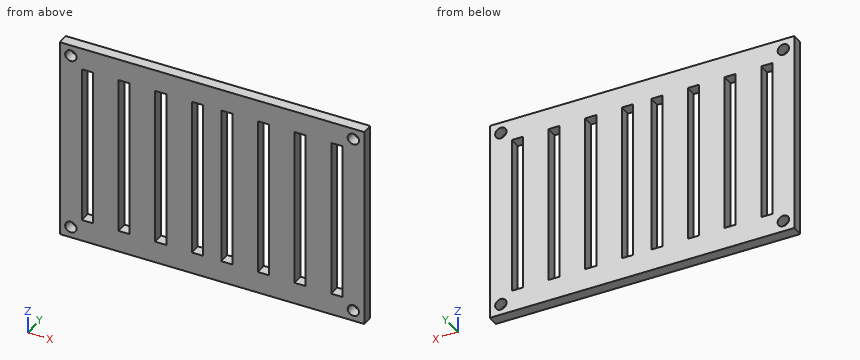
from build123d import *

# Parameters (mm, degrees)
SKETCH_1_W          = 83
SKETCH_1_H          = 56
SKETCH_1_R          = 1.55
EXTRUDE_1_DEPTH     = 3
SKETCH_3_W          = 3
SKETCH_3_H          = 44
CUT_EXTRUDE_1_DEPTH = 51.152268144


with BuildPart() as part:
    # ｽｹｯﾁ1 → ﾎﾞｽ - 押し出し1 (new body)
    with BuildSketch(Plane(origin=(0, 0, 0), x_dir=(1, 0, 0), z_dir=(0, 1, 0))):
        Rectangle(SKETCH_1_W, SKETCH_1_H)
        with Locations(Location((-38.5, 25, 0), (0, 0, 270))):
            Circle(SKETCH_1_R, mode=Mode.SUBTRACT)
        with Locations(Location((38.5, 25, 0), (0, 0, 270))):
            Circle(SKETCH_1_R, mode=Mode.SUBTRACT)
        with Locations(Location((38.5, -25, 0), (0, 0, 270))):
            Circle(SKETCH_1_R, mode=Mode.SUBTRACT)
        with Locations(Location((-38.5, -25, 0), (0, 0, 270))):
            Circle(SKETCH_1_R, mode=Mode.SUBTRACT)
    extrude(amount=EXTRUDE_1_DEPTH)

    # ｽｹｯﾁ3 → ｶｯﾄ - 押し出し1 (cut, through all)
    with BuildSketch(Plane(origin=(0, 3, 0), x_dir=(1, 0, 0), z_dir=(0, 1, 0))):
        with Locations((-34, 0)):
            Rectangle(SKETCH_3_W, SKETCH_3_H)
        with Locations((-24, 0)):
            Rectangle(SKETCH_3_W, SKETCH_3_H)
        with Locations((-14, 0)):
            Rectangle(SKETCH_3_W, SKETCH_3_H)
        with Locations((-4, 0)):
            Rectangle(SKETCH_3_W, SKETCH_3_H)
        with Locations((4, 0)):
            Rectangle(SKETCH_3_W, SKETCH_3_H)
        with Locations((14, 0)):
            Rectangle(SKETCH_3_W, SKETCH_3_H)
        with Locations((24, 0)):
            Rectangle(SKETCH_3_W, SKETCH_3_H)
        with Locations((34, 0)):
            Rectangle(SKETCH_3_W, SKETCH_3_H)
    extrude(amount=-CUT_EXTRUDE_1_DEPTH, mode=Mode.SUBTRACT)


solid = part.part
Can you work these out from the model? Positions are in its coordinate system, mm. Round coordinates to 2 decimals unless told otherwise and drop trailing zeros. Write each loop counter-clockwise with the first axis right and the second up, starting at its lowest first coordinate (ties: lowest second). Pieces come first, ordered by that corner, then holes. Notation, with made-up numbers: (27, 21.5) -> (58, 21.5) arc R23 ccw to (58, 39.5) -> close; hole circle Ø6 at (-7, 56). An arc over 180 degrees is marked (long way). Use one line per item in the form item = value. Start each with the question number.
Q1. Imagine slicing it at C-C (z = 4.5). Count the separate pieces of the cut face and the enclosed holes in it, then the cut area to 3 significant figures.
Q2. Imagine slicing it at A-A (x = -38.5). Please give me the cut outline in (y, z).
Q3. Imagine slicing it at B-B (z = 25). Please give me the cut outline in (x, y), then the cut area to 3 significant figures.
Q4. If I drill on probe 1 along X at (y, z) = (2.4, -25); probe 2 along Z at (x, y) = (25, 2.7), over which ranges is the centre line in solid material (lowest first)? Write a range as [from, to].
Worked out:
q1.separate_pieces = 9
q1.enclosed_holes = 0
q1.area = 177 mm^2
q2.outline = (0, -28) -> (3, -28) -> (3, -26.55) -> (0, -26.55) -> close; (0, -23.45) -> (3, -23.45) -> (3, 23.45) -> (0, 23.45) -> close; (0, 26.55) -> (3, 26.55) -> (3, 28) -> (0, 28) -> close
q3.outline = (-41.5, 0) -> (-40.05, 0) -> (-40.05, 3) -> (-41.5, 3) -> close; (-36.95, 0) -> (36.95, 0) -> (36.95, 3) -> (-36.95, 3) -> close; (40.05, 0) -> (41.5, 0) -> (41.5, 3) -> (40.05, 3) -> close
q3.area = 230 mm^2
q4.probe_1 = [-41.5, -40.05], [-36.95, 36.95], [40.05, 41.5]
q4.probe_2 = [-28, -22], [22, 28]
